Part model, mm, in its own coordinate system. Face numbers are marked on the shaded views. A direction names the side the tool comes from. Give positions to 0.01 mm unless a question says otherwise; leave off trailing zeros. Order: outer loops, then holes, each group sorted by start corner. A loop starts at its lowest first (then second) coordinate and runs counter-clockwise, first axis right, second up. Notation, with made-up numbers: M 35,50 L 74,50 A37 ccw 74,86 Z; hole C -37,38 d11. An arc over 180 degrees is marked long. Answer as a JSON object with one key per item and string values.
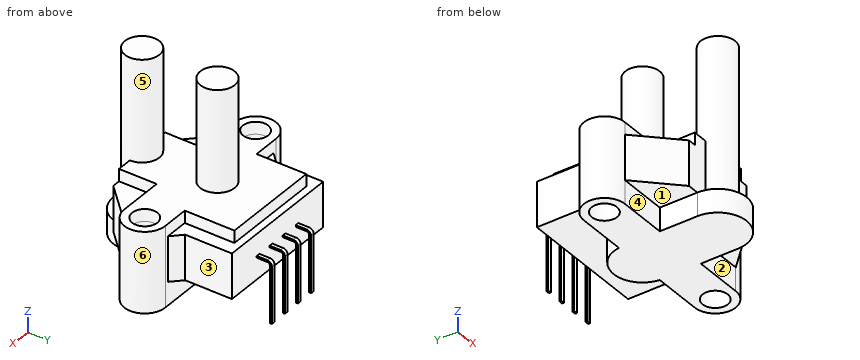
from build123d import *

# Parameters (mm, degrees)
SKETCH1_R           = 1.75
BOSS_EXTRUDE1_DEPTH = 3.25
BOSS_EXTRUDE3_START = -3.25
SKETCH1_4_R         = 1.75
BOSS_EXTRUDE3_DEPTH = 6.25
SKETCH3_W           = 9
SKETCH3_H           = 5.235
SKETCH3_R           = 1.75
SKETCH3_W_2         = 14
SKETCH3_H_2         = 6.925
BOSS_EXTRUDE4_DEPTH = 1.7
SKETCH1_5_R         = 2.4
BOSS_EXTRUDE5_DEPTH = 25.3
SKETCH5_W           = 0.51
SKETCH5_H           = 0.25
LPATTERN1_COUNT     = 4
LPATTERN1_PITCH     = 2.54


with BuildPart() as part:
    # Sketch1 → Boss-Extrude1 (new body)
    with BuildSketch(Plane(origin=(0, 0, 0), x_dir=(1, 0, 0), z_dir=(0, 0, -1))):
        with BuildLine():
            Line((-14.61, 9.925), (-7.785169808, 9.925))
            ThreePointArc((-7.785169808, 9.925), (-3.81, 6.37), (0.165169808, 9.925))
            Line((0.165169808, 9.925), (6.99, 9.925))
            ThreePointArc((6.99, 9.925), (9.845, 12.78), (6.99, 15.635))
            Line((6.99, 15.635), (0.19, 15.635))
            Line((0.19, 15.635), (0.19, 20.87))
            ThreePointArc((0.19, 20.87), (-3.81, 24.87), (-7.81, 20.87))
            Line((-7.81, 20.87), (-7.81, 15.635))
            Line((-7.81, 15.635), (-14.61, 15.635))
            ThreePointArc((-14.61, 15.635), (-17.465, 12.78), (-14.61, 9.925))
        make_face()
        with Locations(Location((-14.61, 12.78, 0), (0, 0, 180))):
            Circle(SKETCH1_R, mode=Mode.SUBTRACT)
        with Locations(Location((6.99, 12.78, 0), (0, 0, 180))):
            Circle(SKETCH1_R, mode=Mode.SUBTRACT)
    extrude(amount=-BOSS_EXTRUDE1_DEPTH)

    # Sketch1<4> → Boss-Extrude3 (add)
    with BuildSketch(Plane(origin=(0, 0, 0), x_dir=(1, 0, 0), z_dir=(0, 0, -1)).offset(BOSS_EXTRUDE3_START)):
        with BuildLine():
            Line((-12.7, 8.515), (-12.7, 2))
            Line((-12.7, 2), (5.08, 2))
            Line((5.08, 2), (5.08, 8.515))
            Line((5.08, 8.515), (6.49, 9.925))
            Line((6.49, 9.925), (6.99, 9.925))
            ThreePointArc((6.99, 9.925), (9.845, 12.78), (6.99, 15.635))
            Line((6.99, 15.635), (1.814694354, 20.87))
            Line((1.814694354, 20.87), (-9.434694354, 20.87))
            Line((-9.434694354, 20.87), (-14.61, 15.635))
            ThreePointArc((-14.61, 15.635), (-17.465, 12.78), (-14.61, 9.925))
            Line((-14.61, 9.925), (-14.11, 9.925))
            Line((-14.11, 9.925), (-12.7, 8.515))
        make_face()
        with Locations(Location((-14.61, 12.78, 0), (0, 0, 180))):
            Circle(SKETCH1_4_R, mode=Mode.SUBTRACT)
        with Locations(Location((6.99, 12.78, 0), (0, 0, 180))):
            Circle(SKETCH1_4_R, mode=Mode.SUBTRACT)
    extrude(amount=-BOSS_EXTRUDE3_DEPTH)

    # Sketch3 → Boss-Extrude4 (add)
    # profile 1 of 3: a face of its own
    with BuildSketch(Plane.XY.offset(9.5)):
        with Locations((-3.81, -18.2525)):
            Rectangle(SKETCH3_W, SKETCH3_H)
    # profile 2 of 3: a face of its own
    with BuildSketch(Plane.XY.offset(9.5)):
        with BuildLine():
            Line((6.99, -15.635), (-14.61, -15.635))
            ThreePointArc((-14.61, -15.635), (-17.465, -12.78), (-14.61, -9.925))
            Line((-14.61, -9.925), (-14.11, -9.925))
            Line((-14.11, -9.925), (6.49, -9.925))
            Line((6.49, -9.925), (6.99, -9.925))
            ThreePointArc((6.99, -9.925), (9.845, -12.78), (6.99, -15.635))
        make_face()
        with Locations(Location((-14.61, -12.78, 0), (0, 0, 180))):
            Circle(SKETCH3_R, mode=Mode.SUBTRACT)
        with Locations(Location((6.99, -12.78, 0), (0, 0, 180))):
            Circle(SKETCH3_R, mode=Mode.SUBTRACT)
    # profile 3 of 3: a face of its own
    with BuildSketch(Plane.XY.offset(9.5)):
        with Locations((-3.81, -6.4625)):
            Rectangle(SKETCH3_W_2, SKETCH3_H_2)
    extrude(amount=BOSS_EXTRUDE4_DEPTH)

    # Sketch1<5> → Boss-Extrude5 (add)
    with BuildSketch(Plane(origin=(0, 0, 0), x_dir=(1, 0, 0), z_dir=(0, 0, -1))):
        with Locations(Location((-3.81, 20.87, 0), (0, 0, 180))):
            Circle(SKETCH1_5_R)
        with Locations(Location((-3.81, 10.37, 0), (0, 0, 180))):
            Circle(SKETCH1_5_R)
    extrude(amount=-BOSS_EXTRUDE5_DEPTH)

    # Sweep1: sweep along a path in Sketch4
    with BuildLine(Plane(origin=(0, 0, 0), x_dir=(0, 0, -1), z_dir=(1, 0, 0))) as sweep1_path:
        Line((-6.375, -2), (-6.375, -0.5))
        ThreePointArc((-6.375, -0.5), (-6.228553391, -0.146446609), (-5.875, 0))
        Line((-5.875, 0), (0, 0))
        Line((0, 0), (2, 0))
    # Sketch5 → Sweep1 (sweep)
    with BuildSketch(Plane(origin=(0, -2, 0), x_dir=(1, 0, 0), z_dir=(0, 1, 0))):
        with Locations((0, -6.375)):
            Rectangle(SKETCH5_W, SKETCH5_H)
    sweep1 = sweep(path=sweep1_path.line)

    # LPattern1: Sweep1 ×4
    with Locations(*[(-i * LPATTERN1_PITCH, 0, 0) for i in range(1, LPATTERN1_COUNT)]):
        add(sweep1)


solid = part.part
1. Cut at B-B on z = 7.25. Give the cut face in (x, y) (3 decimals), plus the area to 3 significant figures.
Worked answers:
{"outline": "M -14.61,-15.635 L -9.435,-20.87 L -6.21,-20.87 A2.4 ccw -1.41,-20.87 L 1.815,-20.87 L 6.99,-15.635 A2.855 ccw 6.99,-9.925 L 6.49,-9.925 L 5.08,-8.515 L 5.08,-2 L -12.7,-2 L -12.7,-8.515 L -14.11,-9.925 L -14.61,-9.925 A2.855 ccw Z; hole C -14.61,-12.78 d3.5; hole C 6.99,-12.78 d3.5", "area": "368 mm^2"}
2. Pin check, flat tips, straight feed: P1, Ø1.5, axis at x = -13.5, y = -2.5, coming from the -Z side; P2, Ø0.5, axis at y = 0, z = 6, coming from the +X side (3 decimals); P3, Ø5, axis at x = -13.5, y = -4.5, coming from the +Z side; P4, Ø6, axis at y = -21, z = 19, coming from the +X side. Stop position of each tip, or through.
Worked answers:
{"P1": "passes through", "P2": "stops at x = 0.255", "P3": "stops at z = 9.5", "P4": "stops at x = -1.41"}
3. Which spindle directions (+Z, -Z, +X, -X, +Y, -Y) get a long thin tool onto all of the face, cutting with end or side? Do the marked faces 1, 2 and 3. Say none if no direction does.
Worked answers:
{"face 1": "-Z, -X, -Y", "face 2": "-Z, +X, -Y", "face 3": "+Z, -Z, +X, +Y"}
4. Two-plate mould, pull along Y, no slides. Class the marked faces 4, 5 and 6: +Y half, -Y half, draft (parallel to the pull), parting line (faces both ways), or undercut.
Worked answers:
{"face 4": "-Y half", "face 5": "undercut", "face 6": "parting line"}
5. Probe line 1 along X through (y, z) = (-12.78, 10.5) (3 decimals); line 2 along Y through (x, z) = (6.99, 4.5) (3 decimals); line 3 along Z through (x, y) = (-5, -2.5). List the from-to ranges inside material, lowest first.
Worked answers:
{"line 1": "x = -17.465 to -16.36, -12.86 to 5.24, 8.74 to 9.845", "line 2": "y = -15.635 to -14.53, -11.03 to -9.925", "line 3": "z = 3.25 to 9.5"}
6. Cut at A-A on z = 2.5. Give the cut face in (x, y) (3 decimals), plus the area to 3 significant figures.
Worked answers:
{"outline": "M -14.61,-15.635 L -7.81,-15.635 L -7.81,-20.87 A4 ccw 0.19,-20.87 L 0.19,-15.635 L 6.99,-15.635 A2.855 ccw 6.99,-9.925 L 0.165,-9.925 A4 ccw -7.785,-9.925 L -14.61,-9.925 A2.855 ccw Z; M -7.875,-0.125 L -7.365,-0.125 L -7.365,0.125 L -7.875,0.125 Z; M -5.335,-0.125 L -4.825,-0.125 L -4.825,0.125 L -5.335,0.125 Z; M -2.795,-0.125 L -2.285,-0.125 L -2.285,0.125 L -2.795,0.125 Z; M -0.255,-0.125 L 0.255,-0.125 L 0.255,0.125 L -0.255,0.125 Z; hole C -14.61,-12.78 d3.5; hole C 6.99,-12.78 d3.5", "area": "219 mm^2"}
7. Cut at C-C on x = -3.81. Give the cut face in (y, z).
Worked answers:
{"outline": "M -24.87,0 L -6.37,0 L -6.37,3.25 L -2,3.25 L -2,9.5 L -3,9.5 L -3,11.2 L -7.97,11.2 L -7.97,25.3 L -12.77,25.3 L -12.77,11.2 L -18.47,11.2 L -18.47,25.3 L -23.27,25.3 L -23.27,3.25 L -24.87,3.25 Z"}
8. Cut at D-D on x = 8. Give the cut face in (y, z), plus the area to 3 significant figures.
Worked answers:
{"outline": "M -15.45,0 L -14.21,0 L -14.21,11.2 L -15.45,11.2 Z; M -11.35,0 L -10.11,0 L -10.11,11.2 L -11.35,11.2 Z", "area": "27.8 mm^2"}
